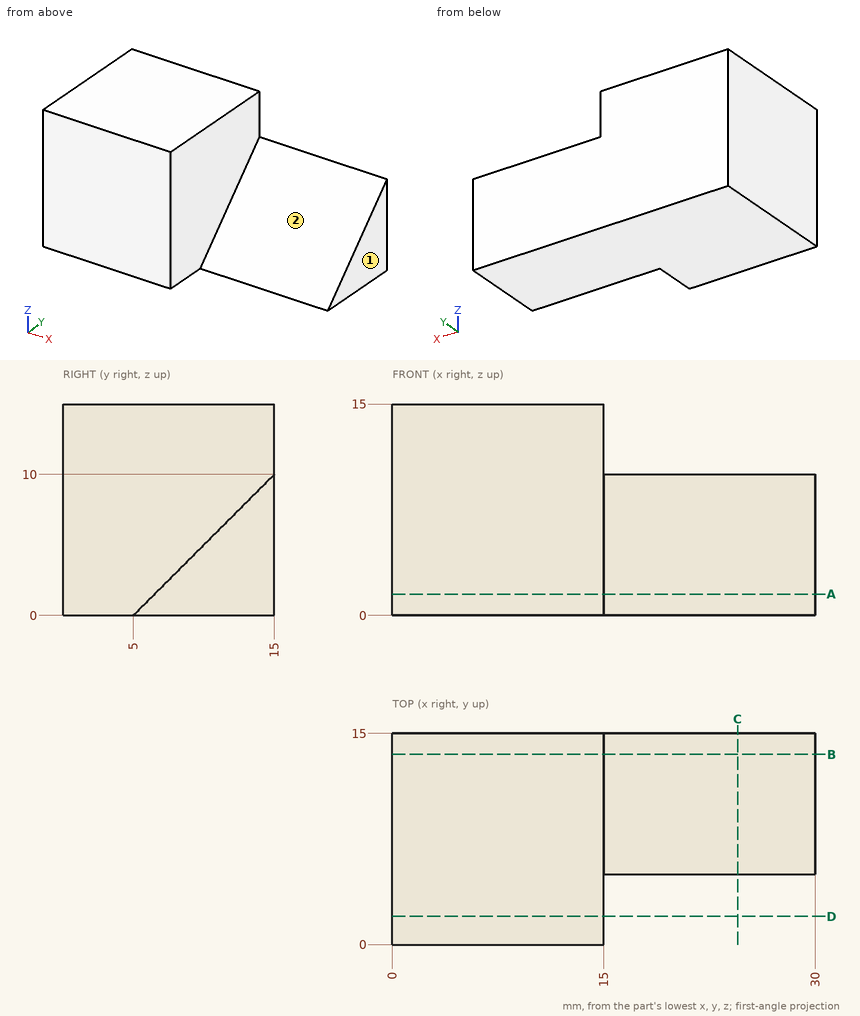
Source: three-view drawing plus pictorial views. Frame: mm from the lowest corner of the part. A direction names the side the tool comes from. Round coordinates to 2 decimals unless told otherwise and drop trailing zeros. Loops run counter-clockwise (first coordinate to the right, second up) from the corner with the lowest first, then second, coordinate; pieces in that order, holes last.
Q1. Section B-B, the plane y = 13.5. Return loops of the section in (x, z).
Q2. Ray query, line 1 (X direction, y = 14, z = 14.5); line 2 (Y direction, x = 16.75, z = 5); line 3 (Z direction, x = 18.25, y = 13). Return the intervals inside material, ascending.
Q3. Access query for the marked faces 1 and 2. Directions: +Z, -Z, +X, -X, +Y, -Y. A direction counts if a zero-diameter tool reaches every point of the face in a straight line with its end or side. Return the directions, or none.
Q4. Section C-C, the plane x = 24.5. Return loops of the section in (y, z).
Q5. First-contact query: P1, Ø3, axis at x = 22.5, y = 9.5, coming from the +Z side; P2, Ø1, axis at x = 26.5, z = 2.5, coming from the -Y side. Flat tips, straight axial feed; report the tip coordinate or a pass-through.
Q6. Section A-A, the plane z = 1.5. Return loops of the section in (x, y), plus the area to 4 significant figures.
Q7. Section D-D, the plane y = 2. Return loops of the section in (x, z).
Solutions:
1. outline: (0, 0) - (30, 0) - (30, 8.5) - (15, 8.5) - (15, 15) - (0, 15) - close
2. line 1: x = 0 to 15
2. line 2: y = 10 to 15
2. line 3: z = 0 to 8
3. face 1: +Z, -Z, +X, +Y, -Y
3. face 2: +Z, +X, -Y
4. outline: (5, 0) - (15, 0) - (15, 10) - close
5. P1: stops at z = 6
5. P2: stops at y = 7
6. outline: (0, 0) - (15, 0) - (15, 6.5) - (30, 6.5) - (30, 15) - (0, 15) - close
6. area: 352.5 mm2
7. outline: (0, 0) - (15, 0) - (15, 15) - (0, 15) - close
